```python
from build123d import *

# Parameters (mm, degrees)
EXTRUDE_1_DEPTH     = 2
SKETCH_3_R          = 1.4
CUT_EXTRUDE_1_DEPTH = 2
SKETCH_4_R          = 9
EXTRUDE_2_DEPTH     = 42


with BuildPart() as part:
    # 草图1 → 凸台-拉伸1 (new body)
    with BuildSketch(Plane.XY):
        Polygon((46.5, 12), (23.5, 35), (-46.5, 35), (-46.5, -35), (23.5, -35), (46.5, -12), align=None)
    extrude(amount=EXTRUDE_1_DEPTH)

    # 草图3 → 切除-拉伸1 (cut)
    with BuildSketch(Plane.XY.offset(2)):
        with Locations((-22.9, 16.25)):
            Circle(SKETCH_3_R)
        with Locations((37.3, 16.25)):
            Circle(SKETCH_3_R)
        with Locations(Location((37.3, -16.25, 0), (0, 0, 180))):
            Circle(SKETCH_3_R)
        with Locations(Location((-22.9, -16.25, 0), (0, 0, 180))):
            Circle(SKETCH_3_R)
    extrude(amount=-CUT_EXTRUDE_1_DEPTH, mode=Mode.SUBTRACT)

    # 草图4 → 凸台-拉伸2 (add)
    with BuildSketch(Plane.XY.offset(2)):
        with Locations(Location((-35.35, -23.85, 0), (0, 0, 180))):
            Circle(SKETCH_4_R)
        with Locations(Location((-12.05, -23.85, 0), (0, 0, 180))):
            Circle(SKETCH_4_R)
        with Locations(Location((11.25, -23.85, 0), (0, 0, 180))):
            Circle(SKETCH_4_R)
        with Locations(Location((-12.05, 0, 0), (0, 0, 180))):
            Circle(SKETCH_4_R)
        with Locations(Location((11.25, 0, 0), (0, 0, 180))):
            Circle(SKETCH_4_R)
        with Locations(Location((-12.05, 23.85, 0), (0, 0, 180))):
            Circle(SKETCH_4_R)
        with Locations(Location((11.25, 23.85, 0), (0, 0, 180))):
            Circle(SKETCH_4_R)
        with Locations(Location((-35.35, 0, 0), (0, 0, 180))):
            Circle(SKETCH_4_R)
        with Locations(Location((-35.35, 23.85, 0), (0, 0, 180))):
            Circle(SKETCH_4_R)
        with Locations(Location((34.25, 0, 0), (0, 0, 180))):
            Circle(SKETCH_4_R)
    extrude(amount=EXTRUDE_2_DEPTH)


solid = part.part
```
The listing builds one solid part. Answer for the finished solid, in the listing's coordinates (mm). A direction names the side the tool comes from. Give positions to 0.01 mm unless a question says otherwise; leave off trailing zeros. Order: outer loops, then holes, each group sorted by start corner. A loop starts at its lowest first (then second) coordinate and runs counter-clockwise, first axis right, second up. Notation, with made-up numbers: (-10, 14.5) -> (36, 14.5) arc R12 cw to (36, 29.5) -> close; hole circle Ø1 at (75.25, 5). An arc over 180 degrees is marked (long way). One line per item, written item: value.
1) Find section D-D, the plane y = 0. Determine the outline of the cut face in (x, z), plus the area to 3 significant figures.
Reported:
outline: (-46.5, 0) -> (46.5, 0) -> (46.5, 2) -> (43.25, 2) -> (43.25, 44) -> (25.25, 44) -> (25.25, 2) -> (20.25, 2) -> (20.25, 44) -> (2.25, 44) -> (2.25, 2) -> (-3.05, 2) -> (-3.05, 44) -> (-21.05, 44) -> (-21.05, 2) -> (-26.35, 2) -> (-26.35, 44) -> (-44.35, 44) -> (-44.35, 2) -> (-46.5, 2) -> close
area: 3,210 mm^2
2) Find section C-C, the plane x = -12.05. Determine the outline of the cut face in (y, z), plus the area to 3 significant figures.
Reported:
outline: (-35, 0) -> (35, 0) -> (35, 2) -> (32.85, 2) -> (32.85, 44) -> (14.85, 44) -> (14.85, 2) -> (9, 2) -> (9, 44) -> (-9, 44) -> (-9, 2) -> (-14.85, 2) -> (-14.85, 44) -> (-32.85, 44) -> (-32.85, 2) -> (-35, 2) -> close
area: 2,410 mm^2
3) Determine the mould class of faces 1 (the cylindrical face through (43.24, -0.4, 22.71)), 2 (the cylindrical face through (-10.878, -32.773, 22.706)), 3 (the flat face through (-35, 0, 44)) for opening direction Y: pulls with the +Y half, pulls with the -Y half, needs draft (parallel to the pull), parting line crosses it, or undercut.
Reported:
face 1: parting line crosses it
face 2: undercut
face 3: needs draft
4) Find the intervals of material crossed by line 1 (X direction, y = -24, z = 39); line 2 (Y direction, x = -22.9, z = 0.6); line 3 (Y direction, x = -30.5, z = 10), in increasing order.
Reported:
line 1: x = -44.35 to -26.35, -21.05 to -3.05, 2.25 to 20.25
line 2: y = -35 to -17.65, -14.85 to 14.85, 17.65 to 35
line 3: y = -31.43 to -16.27, -7.58 to 7.58, 16.27 to 31.43
5) Flat-ended cylindrical pins translate along their axes: P1, Ø12, axis at x = 17, z = 9, coming from the -Y side; P2, Ø4, axis at x = -28.5, z = 16.5, coming from the -Y side; P3, Ø3, axis at y = -15, z = 17.5, coming from the -X side. Find the tip coordinate at first contact, or state that the pin passes through.
Reported:
P1: stops at y = -32.85
P2: stops at y = -31.43
P3: stops at x = -40.54
6) Find section B-B, the plane y = -16.25. Determine the outline of the cut face in (x, z), plus the area to 3 significant figures.
Reported:
outline: (-46.5, 0) -> (-24.3, 0) -> (-24.3, 2) -> (-30.53, 2) -> (-30.53, 44) -> (-40.17, 44) -> (-40.17, 2) -> (-46.5, 2) -> close; (-21.5, 0) -> (35.9, 0) -> (35.9, 2) -> (16.07, 2) -> (16.07, 44) -> (6.43, 44) -> (6.43, 2) -> (-7.23, 2) -> (-7.23, 44) -> (-16.87, 44) -> (-16.87, 2) -> (-21.5, 2) -> close; (38.7, 0) -> (42.25, 0) -> (42.25, 2) -> (38.7, 2) -> close
area: 1,380 mm^2
7) Find section A-A, the plane z = 41.5. Count the separate pieces of the cut face and the enclosed holes in it, plus the area to 3 significant figures.
Reported:
separate pieces: 10
enclosed holes: 0
area: 2,540 mm^2
8) A tool of negligible diameter and unlimited length cuts with its end or side. For faces 4 (the flat face through (35.2, 23.3, 1)), 5 (the cylindrical face through (12.422, 14.927, 22.706)), from which of +Z, -Z, +X, -X, +Y, -Y can it reach the whole face along a straight path? Write none if from no direction.
Reported:
face 4: +Z, -Z, +X, +Y
face 5: +Z
